Answer from the drawing. Dimensions are ordinates in mm from the lowest x, y and z of the part. A direction names the side the tool comes from. Coordinates: 2 decimals unless noted, no trailing zeros. Write each loop counter-clockwise with the first axis right and the second up, starting at its lowest first coordinate (ties: lowest second). Pieces come first, ordered by that corner, then holes.
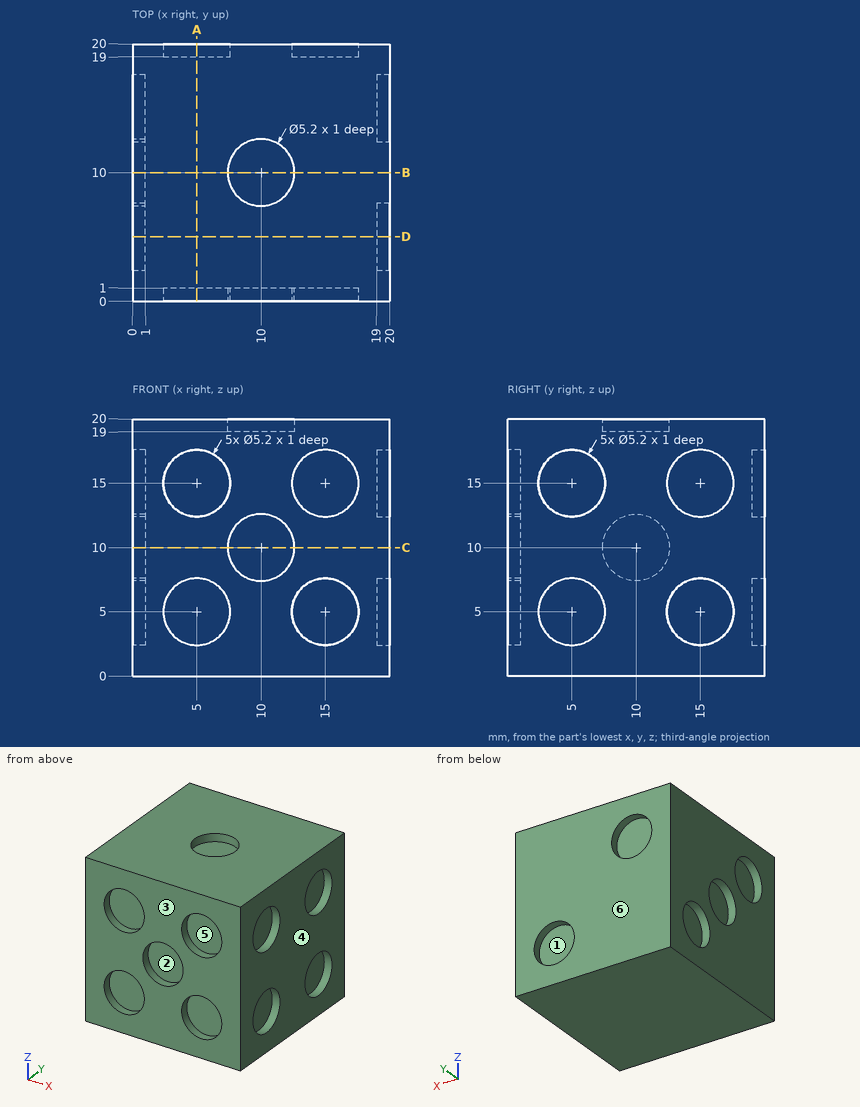
(1) Section C-C, the plane z = 10 is taken. Write down the section's boundary in (x, y).
(2) Section D-D, the plane y = 5 is taken. Write down the section's boundary in (x, z).
(3) Find the intervals of material crossed by probe 1 along Z at (x, y) = (19.7, 5); probe 2 along Z at (x, y) = (5, 19.85); probe 3 along X at (y, z) = (16.5, 5.5), in increasing order.
(4) Which of the six approach directions +Z, -Z, +X, -X, +Y, -Y give full straight-line access (tool end or side, diameter ignored) to the marked faces 1, 2 and 3?
(5) Each of these flat-tipped pins is pushed along its axis until it touches: pin 1 (3 mm diameter, centred on y = 5, z = 15, fed in from -X); pin 2 (4 mm diameter, centred on x = 15, z = 15, fed in from -Y); pin 3 (6 mm diameter, centred on x = 4, z = 12, fed in from -Y); pin 4 (1.6 mm diameter, centred on y = 16, z = 4.5, fed in from +X). Where does it stop, or does it pass through?
(6) Section B-B, the plane y = 10 is taken. Write down the section's boundary in (x, z), plus the area to 3 significant figures.
(7) For a pull along X with two mould halves and no side action, classify the marked faces 4, 5 and 6 as pulls with the +X half, pulls with the -X half, needs draft (parallel to the pull), parting line crosses it, or undercut.
(8) Section A-A, the plane x = 5 is taken. Write down the section's boundary in (y, z).
Solution:
1. outline: (0, 0) - (7.4, 0) - (7.4, 1) - (12.6, 1) - (12.6, 0) - (20, 0) - (20, 20) - (0, 20) - (0, 12.6) - (1, 12.6) - (1, 7.4) - (0, 7.4) - close
2. outline: (0, 0) - (20, 0) - (20, 2.4) - (19, 2.4) - (19, 7.6) - (20, 7.6) - (20, 12.4) - (19, 12.4) - (19, 17.6) - (20, 17.6) - (20, 20) - (0, 20) - (0, 17.6) - (1, 17.6) - (1, 12.4) - (0, 12.4) - close
3. probe 1: z = 0 to 2.4, 7.6 to 12.4, 17.6 to 20
3. probe 2: z = 0 to 12.4, 17.6 to 20
3. probe 3: x = 1 to 19
4. face 1: +Y
4. face 2: -Y
4. face 3: +Z, -Z, +X, -X, -Y
5. pin 1: stops at x = 1
5. pin 2: stops at y = 1
5. pin 3: stops at y = 0
5. pin 4: stops at x = 19
6. outline: (0, 0) - (20, 0) - (20, 20) - (12.6, 20) - (12.6, 19) - (7.4, 19) - (7.4, 20) - (0, 20) - (0, 12.6) - (1, 12.6) - (1, 7.4) - (0, 7.4) - close
6. area: 390 mm2
7. face 4: pulls with the +X half
7. face 5: undercut
7. face 6: needs draft
8. outline: (0, 0) - (20, 0) - (20, 12.4) - (19, 12.4) - (19, 17.6) - (20, 17.6) - (20, 20) - (0, 20) - (0, 17.6) - (1, 17.6) - (1, 12.4) - (0, 12.4) - (0, 7.6) - (1, 7.6) - (1, 2.4) - (0, 2.4) - close
